Here's how the part is built. I have some questions about the finished solid (model axes, mm). Give positions to 0.01 mm unless a question says otherwise; leave off trailing zeros. Write each loop counter-clockwise with the first axis right and the second up, starting at its lowest first coordinate (ties: lowest second). Pieces come first, ordered by that corner, then holes. Notation, with made-up numbers: (8, 88.5) -> (50, 88.5) arc R13 cw to (50, 113.5) -> close; hole circle Ø10 at (-40, -23). An arc over 180 degrees is marked (long way). Use CSV: the item, a comma, the result in double quotes. Start each with the question number.
(1) Suppose I cut it at A-A on x = -48. List the corners of the cut face in (y, z) for me, plus the area to 3 significant figures.
(2) For pin 1 Ø1.5 at (y, z) = (23, 0.5) entering from -X; pin 2 Ø1.3 at (x, z) = (-63.5, 1.5) entering from +Y; pin 3 Ø2 at (y, z) = (-219, 2.5) entering from -X (3 decimals), each with a flat end and sliding along its axis, tell me the tip position at first contact or that it passes through.
(3) I need wall thicknesses on L1, parallel to Y at x = 5.5, z = 3.95; L2, parallel to X at y = 199, z = 4.15. Which ranges of each line are inside material? Lowest first, please. Write a range as [from, to].
from build123d import *

# Parameters (mm, degrees)
SKETCH1_W           = 130.175
SKETCH1_H           = 431.8
BOSS_EXTRUDE1_DEPTH = 4.3434
SKETCH2_W           = 8.6868
SKETCH2_H           = 19.05
SKETCH2_W_2         = 19.05
SKETCH2_H_2         = 8.6868
CUT_EXTRUDE1_DEPTH  = 226.539481643
SKETCH3_W           = 19.05
SKETCH3_H           = 8.6868
BOSS_EXTRUDE2_DEPTH = 4.3434


with BuildPart() as part:
    # Sketch1 → Boss-Extrude1 (new body)
    with BuildSketch(Plane.XY):
        Rectangle(SKETCH1_W, SKETCH1_H)
    extrude(amount=BOSS_EXTRUDE1_DEPTH)

    # Sketch2 → Cut-Extrude1 (cut, through all)
    with BuildSketch(Plane.XY.offset(4.3434)):
        with Locations((-65.0875, 190.5)):
            Rectangle(SKETCH2_W, SKETCH2_H)
        with Locations((-25.4, 215.9)):
            Rectangle(SKETCH2_W_2, SKETCH2_H_2)
        with Locations((25.4, 215.9)):
            Rectangle(SKETCH2_W_2, SKETCH2_H_2)
        with Locations((-65.0875, 136.398)):
            Rectangle(SKETCH2_W, SKETCH2_H)
        with Locations((-65.0875, 82.296)):
            Rectangle(SKETCH2_W, SKETCH2_H)
        with Locations((-65.0875, 28.194)):
            Rectangle(SKETCH2_W, SKETCH2_H)
    cut_extrude1 = extrude(amount=-CUT_EXTRUDE1_DEPTH, mode=Mode.SUBTRACT)

    # Mirror1: Cut-Extrude1 across plane
    add(cut_extrude1.mirror(Plane.ZX), mode=Mode.SUBTRACT)

    # Sketch3 → Boss-Extrude2 (add)
    with BuildSketch(Plane.XY):
        with Locations((-25.4, 215.9)):
            Rectangle(SKETCH3_W, SKETCH3_H)
        with Locations((25.4, 215.9)):
            Rectangle(SKETCH3_W, SKETCH3_H)
    boss_extrude2 = extrude(amount=BOSS_EXTRUDE2_DEPTH)

    # Mirror2: Boss-Extrude2 across plane
    add(boss_extrude2.mirror(Plane.ZX))


solid = part.part
Geometry says:
1,outline,"(-215.9, 0) -> (215.9, 0) -> (215.9, 4.34) -> (-215.9, 4.34) -> close"
1,area,"1,880 mm²"
2,pin 1,"x = -60.74"
2,pin 2,"y = 215.9"
2,pin 3,"x = -34.925"
3,L1,"[-215.9, 215.9]"
3,L2,"[-60.74, 65.09]"
